Can you work these out from the drawing? Everything is in mm from the part's minimum corner. A direction names the side the tool comes from. Give positions to 0.01 mm unless a question says otherwise; leave off trailing zeros. Loops run counter-clockwise (first coordinate to the right, second up) from the corner with the lowest first, then second, coordinate; pieces in that order, holes last. Notation, with made-up numbers: (-17.75, 70.25) - (28.25, 70.25) arc R21 cw to (28.25, 75.25) - close; hole circle Ø10 at (26.25, 5.25). An arc over 180 degrees is marked (long way). One line per item, written item: value. Start each with the question number.
Q1. For the marked faces 4, 5, 6 and 7, which set-ups out of +Z, -Z, +X, -X, +Y, -Y let a thin tool reach every point of the face, with its end or its side?
Q2. I want a section at C-C (z = 125). Please give me the cut outline in (x, y), then the cut area to 3 significant figures.
Q3. If I drill on line 1 (Y direction, x = 89, z = 120.5); line 2 (Z direction, x = 40, y = 409); line 3 (Y direction, x = 44, z = 227.5), over which ranges is the centre line in solid material (lowest first)? Write a range as from..to.
Q4. I want a section at B-B (x = 94.5). Please give me the cut outline in (y, z), then the cut area to 3 significant figures.
Q5. I want a section at A-A (z = 154). Please give me the cut outline in (x, y), then the cut area to 3 significant figures.
Q6. I'm going to push flat-ended pins straight in: P1, Ø5, axis at x = 118, y = 136.5, coming from the -Z side; P2, Ø5, axis at x = 96, y = 346.5, coming from the +Z side; P3, Ø12, axis at x = 72, y = 363, coming from the +Z side; P4, Ø5, axis at y = 381.5, z = 124, coming from the +X side. Where does each tip first touch, or does it pass through?
Q7. I want a section at D-D (x = 75). Please give me the cut outline in (y, z), then the cut area to 3 significant figures.
Q8. If we mould it in two halves opening along Y, with no side actions, what happens to the marked faces 1, 2 and 3? For each: released by +Y, released by -Y, zero draft, split by the parting line, or undercut.
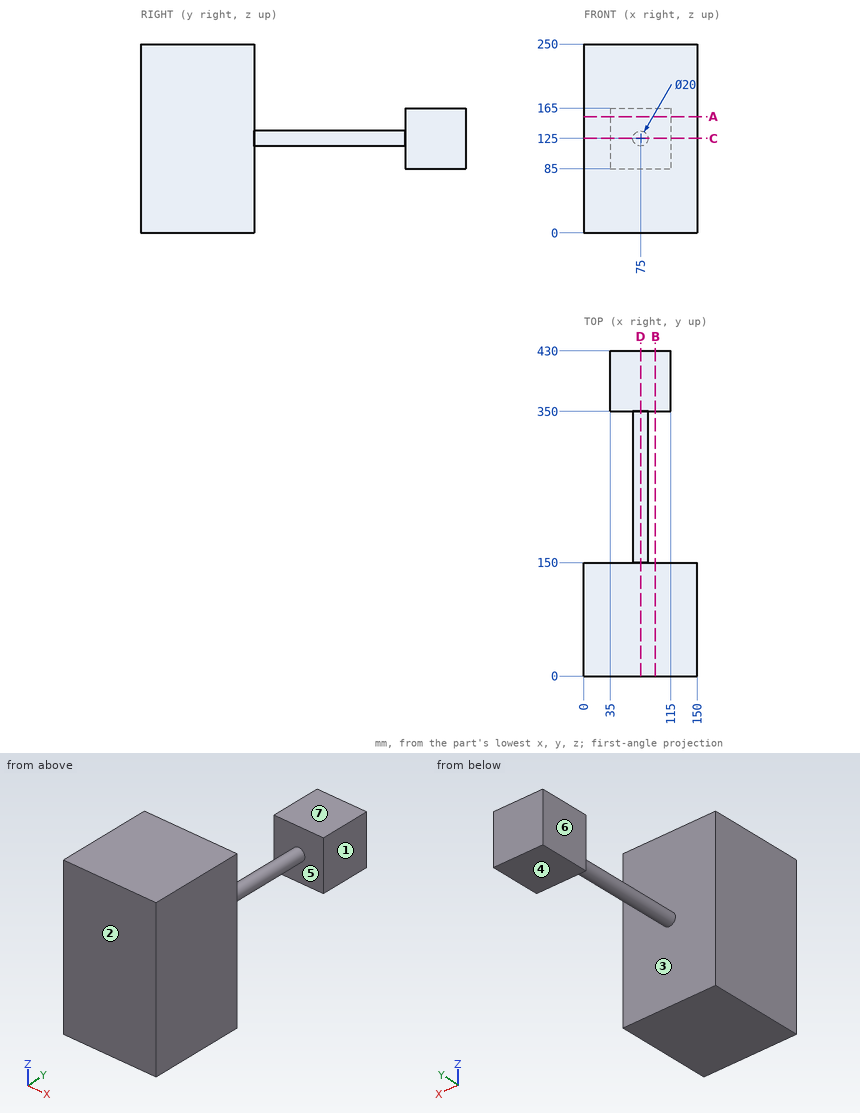
Worked answers:
1. face 4: -Z, +X, -X, +Y
1. face 5: none
1. face 6: +Z, -Z, -X, +Y
1. face 7: +Z, +X, -X, +Y
2. outline: (0, 0) - (150, 0) - (150, 150) - (85, 150) - (85, 350) - (115, 350) - (115, 430) - (35, 430) - (35, 350) - (65, 350) - (65, 150) - (0, 150) - close
2. area: 32,900 mm²
3. line 1: y = 0..150, 350..430
3. line 2: z = 85..165
3. line 3: y = 0..150
4. outline: (0, 0) - (150, 0) - (150, 250) - (0, 250) - close; (350, 85) - (430, 85) - (430, 165) - (350, 165) - close
4. area: 43,900 mm²
5. outline: (0, 0) - (150, 0) - (150, 150) - (0, 150) - close; (35, 350) - (115, 350) - (115, 430) - (35, 430) - close
5. area: 28,900 mm²
6. P1: stops at z = 0
6. P2: passes through
6. P3: stops at z = 165
6. P4: stops at x = 115
7. outline: (0, 0) - (150, 0) - (150, 115) - (350, 115) - (350, 85) - (430, 85) - (430, 165) - (350, 165) - (350, 135) - (150, 135) - (150, 250) - (0, 250) - close
7. area: 47,900 mm²
8. face 1: zero draft
8. face 2: released by -Y
8. face 3: undercut
